For this review, take the finished solid that the model builds, in its own axes (mm). A direction names the side the tool comes from. Coordinates: 2 decimals unless noted, no trailing zeros. Write each loop counter-clockwise with the first axis right and the second up, starting at its lowest first coordinate (ties: lowest second). Pieces come first, ordered by that corner, then holes. Notation, with made-up numbers: (8.25, 23.25) -> (47.25, 23.25) arc R18 cw to (47.25, 39.25) -> close; hole circle Ø2 at (8.5, -37.5). An arc over 180 degrees is marked (long way). One line per item, written item: value. Start each with the question number.
1) Add section B-B (z = -8). State the section outline as (x, y) points (3 decimals).
2) For probe 1 along Z at (x, y) = (30.5, 28.5) (3 decimals); probe 2 along X at (y, z) = (0.5, 11); probe 3 along Y at (x, z) = (31, -11) (3 decimals), list the stretches that pass through material, from the lowest coordinate up. Write a range as from..to.
3) Add section A-A (x = 24). State the section outline as (y, z) points (3 decimals), and give its area (3 significant figures).
4) Machinability: for faces 1 (the cylindrical face through (3.086, -0.86, -9.955)), 2 (the flat face through (22, 15, 9.525)), 3 (the flat face through (22, 15, 0)), 4 (the flat face through (47.625, -2, 5)), which of the approach directions +Z, -Z, +X, -X, +Y, -Y give a long, thin tool a straight path to every point of the face, cutting with its end or side? Answer none if there is none.
5) Mouldability with a two-part tool opening along Z and no side actions: class faces 5 (the cylindrical face through (3.086, -0.86, 15.445)), 6 (the cylindrical face through (21.87, 3.33, -1.91)), 7 (the flat face through (-3.175, -2, 5)) as released by +Z, released by -Z, zero draft, split by the parting line, or undercut.
6) Add section D-D (x = 10.5). State the section outline as (y, z) points (3 decimals).
7) For pin 1 Ø5.5 at (x, z) = (41.28, -7.94) entering from +Y; pin 2 Ø3 at (x, z) = (10, 18) entering from +Y; pin 3 Ø10 at (x, z) = (4, 0.5) entering from +Y; pin 4 Ø6.5 at (x, y) = (22.22, 20.84) entering from +Z, all flat-tipped, find the tip position at first contact; note any pin that passes through.
from build123d import *

# Parameters (mm, degrees)
SKETCH1_R                       = 5.55625
BOSS_EXTRUDE1_DEPTH             = 9.525
BOSS_EXTRUDE2_DEPTH             = 12.7
CHAMFER3_SIZE                   = 2.54
BOSS_EXTRUDE3_START             = 12.7
BOSS_EXTRUDE3_DEPTH             = 12.7
CHAMFER4_SIZE                   = 2.54
FILLET4_R                       = 6.35
SKETCH9_W                       = 2.0193
SKETCH9_H                       = 4.6961896
F_10_32_TAPPED_HOLE1_AT_2_COUNT = 2
F_10_32_TAPPED_HOLE1_AT_2_PITCH = 38.1
F_10_32_TAPPED_HOLE1_AT_3_COUNT = 2
F_10_32_TAPPED_HOLE1_AT_3_PITCH = 45.790501198
F_10_32_TAPPED_HOLE1_AT_4_COUNT = 2
F_10_32_TAPPED_HOLE1_AT_4_PITCH = 25.4


with BuildPart() as part:
    # Sketch1 → Boss-Extrude1 (new body)
    with BuildSketch(Plane.XY):
        with BuildLine():
            Line((0, -3.175), (44.45, -3.175))
            Line((44.45, -3.175), (47.625, -3.175))
            Line((47.625, -3.175), (47.625, 0))
            ThreePointArc((47.625, 0), (47.52643593, 0.784963037), (47.236863327, 1.5211896))
            Line((47.236863327, 1.5211896), (33.372453307, 26.9211896))
            ThreePointArc((33.372453307, 26.9211896), (22.225, 33.536431201), (11.077546693, 26.9211896))
            Line((11.077546693, 26.9211896), (-2.786863327, 1.5211896))
            ThreePointArc((-2.786863327, 1.5211896), (-3.07643593, 0.784963037), (-3.175, 0))
            Line((-3.175, 0), (-3.175, -3.175))
            Line((-3.175, -3.175), (0, -3.175))
        make_face()
        with Locations(Location((22.225, 20.836431201, 0), (0, 0, 180))):
            Circle(SKETCH1_R, mode=Mode.SUBTRACT)
    extrude(amount=BOSS_EXTRUDE1_DEPTH)

    # Sketch4 → Boss-Extrude2 (add)
    with BuildSketch(Plane.XY.offset(9.525)):
        with BuildLine():
            Line((47.625, -3.175), (47.625, 0))
            ThreePointArc((47.625, 0), (47.52643593, 0.784963037), (47.236863327, 1.5211896))
            Line((47.236863327, 1.5211896), (-2.786863327, 1.5211896))
            ThreePointArc((-2.786863327, 1.5211896), (-3.07643593, 0.784963037), (-3.175, 0))
            Line((-3.175, 0), (-3.175, -3.175))
            Line((-3.175, -3.175), (47.625, -3.175))
        make_face()
    extrude(amount=BOSS_EXTRUDE2_DEPTH)

    # Chamfer3
    chamfer3_edges = [part.edges().sort_by_distance(p)[0] for p in [
        (22.225, 1.5211896, 22.225),
    ]]
    chamfer(chamfer3_edges, length=CHAMFER3_SIZE)

    # Sketch6 → Boss-Extrude3 (add)
    with BuildSketch(Plane(origin=(0, 0, 0), x_dir=(-1, 0, 0), z_dir=(0, 0, -1)).offset(BOSS_EXTRUDE3_START)):
        with BuildLine():
            Line((3.175, 0), (3.175, -3.175))
            Line((3.175, -3.175), (-47.625, -3.175))
            Line((-47.625, -3.175), (-47.625, 0))
            ThreePointArc((-47.625, 0), (-47.52643593, 0.784963037), (-47.236863327, 1.5211896))
            Line((-47.236863327, 1.5211896), (2.786863327, 1.5211896))
            ThreePointArc((2.786863327, 1.5211896), (3.07643593, 0.784963037), (3.175, 0))
        make_face()
    extrude(amount=-BOSS_EXTRUDE3_DEPTH)

    # Chamfer4
    chamfer4_edges = [part.edges().sort_by_distance(p)[0] for p in [
        (22.225, 1.5211896, -12.7),
    ]]
    chamfer(chamfer4_edges, length=CHAMFER4_SIZE)

    # Fillet4
    fillet4_edges = [part.edges().sort_by_distance(p)[0] for p in [
        (22.225, 1.5211896, 9.525),
        (22.225, 1.5211896, 0),
    ]]
    fillet(fillet4_edges, radius=FILLET4_R)

    # Sketch9 → #10-32 Tapped Hole1 (revolve, cut)
    with BuildSketch(Plane(origin=(3.175, 1.5211896, -7.9375), x_dir=(0, 0, 1), z_dir=(1, 0, 0))):
        with Locations((1.00965, 2.3480948)):
            Rectangle(SKETCH9_W, SKETCH9_H)
    f_10_32_tapped_hole1 = revolve(axis=Axis((3.175, 7.8711896, -7.9375), (0, -1, 0)), mode=Mode.SUBTRACT)

    # #10-32 Tapped Hole1 at 2: #10-32 Tapped Hole1 ×2
    with Locations(*[(i * F_10_32_TAPPED_HOLE1_AT_2_PITCH, 0, 0) for i in range(1, F_10_32_TAPPED_HOLE1_AT_2_COUNT)]):
        add(f_10_32_tapped_hole1, mode=Mode.SUBTRACT)

    # #10-32 Tapped Hole1 at 3: #10-32 Tapped Hole1 ×2
    with Locations(*[Vector(0.8320502943378437, 0, 0.5547001962252291) * (i * F_10_32_TAPPED_HOLE1_AT_3_PITCH) for i in range(1, F_10_32_TAPPED_HOLE1_AT_3_COUNT)]):
        add(f_10_32_tapped_hole1, mode=Mode.SUBTRACT)

    # #10-32 Tapped Hole1 at 4: #10-32 Tapped Hole1 ×2
    with Locations(*[(0, 0, i * F_10_32_TAPPED_HOLE1_AT_4_PITCH) for i in range(1, F_10_32_TAPPED_HOLE1_AT_4_COUNT)]):
        add(f_10_32_tapped_hole1, mode=Mode.SUBTRACT)


solid = part.part
Numbers:
1. outline: (-3.175, -3.175) -> (1.157, -3.175) -> (1.157, 1.521) -> (-2.787, 1.521) arc R3.175 ccw to (-3.175, 0) -> close; (5.193, -3.175) -> (39.257, -3.175) -> (39.257, 1.521) -> (5.193, 1.521) -> close; (43.293, -3.175) -> (47.625, -3.175) -> (47.625, 0) arc R3.175 ccw to (47.237, 1.521) -> (43.293, 1.521) -> close
2. probe 1: 0..9.525
2. probe 2: -3.14..47.59
2. probe 3: -3.175..0.681
3. outline: (-3.175, -12.7) -> (-1.019, -12.7) -> (1.521, -10.16) -> (1.521, -6.35) arc R6.35 cw to (7.871, 0) -> (15.571, 0) -> (15.571, 9.525) -> (7.871, 9.525) arc R6.35 cw to (1.521, 15.875) -> (1.521, 19.685) -> (-1.019, 22.225) -> (-3.175, 22.225) -> close; (26.102, 0) -> (33.412, 0) -> (33.412, 9.525) -> (26.102, 9.525) -> close
3. area: 378 mm²
4. face 1: -Y
4. face 2: +Z, +X, -X, +Y
4. face 3: -Z, +X, -X, +Y
4. face 4: +Z, -Z, +X, +Y, -Y
5. face 5: undercut
5. face 6: released by -Z
5. face 7: zero draft
6. outline: (-3.175, -12.7) -> (-1.019, -12.7) -> (1.521, -10.16) -> (1.521, -6.35) arc R6.35 cw to (7.871, 0) -> (25.863, 0) -> (25.863, 9.525) -> (7.871, 9.525) arc R6.35 cw to (1.521, 15.875) -> (1.521, 19.685) -> (-1.019, 22.225) -> (-3.175, 22.225) -> close
7. pin 1: y = 1.63
7. pin 2: y = 1.52
7. pin 3: y = 23.12
7. pin 4: through
